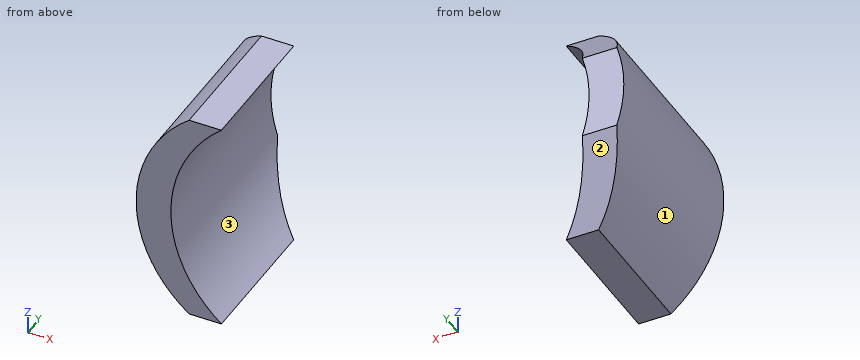
Autodesk Inventor part; units mm, degrees
ref_plane "YZ Plane" through (0, 0, 0) normal (1, 0, 0) x (0, 1, 0)
ref_plane "XZ Plane" through (0, 0, 0) normal (0, 1, 0) x (-1, 0, 0)
ref_plane "XY Plane" through (0, 0, 0) normal (0, 0, 1) x (1, 0, 0)
sketch "Sketch1" plane through (0, 0, 0) normal (0, 1, 0) x (-1, 0, 0)
  arc A0 (0, -6.5) -> (0, 6.5) centre (0, 0) ccw
  line L0 (0, 6.5) -> (0, -6.5)
  dimension "d0" = 13
extrude "Extrusion1" add sketch "Sketch1" along normal blind 12
ref_plane "Work Plane1" through (-10, 0, 6.5) normal (1, 0, 0) x (0, 0, -1)
sketch "Sketch2" plane through (-10, 0, 6.5) normal (1, 0, 0) x (0, 0, -1)
  line L0 (1.5, 8.0057) -> (1.5, 1.5057)
  line L1 (1.5, 1.5057) -> (11.5, 1.5057)
  line L2 (11.5, 1.5057) -> (11.5, 8)
  line L3 (8.5, 10.5) -> (4.5, 10.5)
  line L4 (8.5, 10.5) -> (11.5, 8)
  line L5 (4.5, 10.5) -> (1.5, 8.0057)
  line L6 (13, 0) -> (13, 12)
  point P0 (6.5, 0)
  dimension "d9" = 10
  dimension "d10" = 6.5
  dimension "d12" = 4
  dimension "d14" = 3
  dimension "d15" = 3
  dimension "d24" = 1.5
extrude "Extrusion2" add sketch "Sketch2" along normal blind 10
sketch "Sketch7" plane through (0, 0, 0) normal (0, 1, 0) x (-1, 0, 0)
  arc A0 (0, -6.5) -> (0, 6.5) centre (0, 0) ccw
  line L0 (0, 6.5) -> (0, -6.5)
  line L1 (0, -6.5) -> (0, 6.5)
extrude "Extrusion7" cut sketch "Sketch7" along normal through all
sketch "Sketch8" plane through (0, 0, 0) normal (0, 1, 0) x (-1, 0, 0)
  arc A0 (5.6533, -5) -> (5.6533, 5) centre (1.7994, 0) ccw
  line L0 (5.6533, -5) -> (4.1533, -5)
  line L1 (5.6533, 5) -> (4.1533, 5)
  line L2 (10, 5) -> (4.1533, 5)
  arc A1 (4.1533, -5) -> (4.1533, 5) centre (10.21, 0) ccw
  point P0 (0, 0)
  dimension "d36" = 1.5
  dimension "d37" = 1.5
extrude "Extrusion8" cut sketch "Sketch8" along normal through all both and the other way through all
properties part number "13mm_radius_mold_with_crystal_skull"
CAD build for the part. Positions are in the model's coordinates, mm. Face numbers are marked on the shaded views. Give positions to 0.01 mm unless a question says otherwise; leave off trailing zeros. Order: outer loops, then holes, each group sorted by start corner. A loop starts at its lowest first (then second) coordinate and runs counter-clockwise, first axis right, second up. Notation, with made-up numbers: (65.5, 61.5) - (90.5, 61.5) arc R17 cw to (90.5, 83.5) - close; hole circle Ø9 at (5.5, 74.25). An arc over 180 degrees is marked (long way). Answer in a Markdown table with one row per item.
1. Flat gauge pins, fed straight in: pin 1 (1 mm diameter, centred on x = -6.5, y = 9, fed in from +Z); pin 2 (5 mm diameter, centred on y = 6, z = -4, fed in from -X); pin 3 (5 mm diameter, centred on y = 3, z = -3, fed in from -X). Where does each tip first touch, or does it go through?
Data:
| item | result |
|---|---|
| pin 1 | stops at z = 4.38 |
| pin 2 | stops at x = -7.93 |
| pin 3 | stops at x = -8.09 |
2. Probe probe 1 along Z at (x, y) = (-4.8, 7.75); probe 2 along Z at (x, y) = (-4.55, 4); probe 3 along X at (y, z) = (4.25, -2). List the from-to ranges inside material, lowest first. Write a range as [from, to].
Data:
| item | result |
|---|---|
| probe 1 | z = [-5, -4.38], [4.38, 5] |
| probe 2 | z = [-5, -4.64], [4.64, 5] |
| probe 3 | x = [-7.79, -6.18] |
3. Saw through at D-D, the plane z = 3.25. Give the cut face in (x, y).
Data:
| item | result |
|---|---|
| outline | (-7.21, 1.51) - (-5.63, 1.51) - (-5.63, 9.46) - (-7.21, 9.46) - close |
4. Pull direction Z, two halves, no side cores. Call the marked faces 1, 2 and 3: pulls with the +Z half, pulls with the -Z half, needs draft (parallel to the pull), parting line crosses it, or undercut.
Data:
| item | result |
|---|---|
| face 1 | parting line crosses it |
| face 2 | pulls with the -Z half |
| face 3 | undercut |
5. Saw through at C-C, the plane y = 2. Give the cut face in (x, z), plus the area to 3 significant figures.
Data:
| item | result |
|---|---|
| outline | (-5.65, -5) - (-4.15, -5) arc R6.5 cw to (-4.15, 5) - (-5.65, 5) arc R6.31 ccw to start |
| area | 15.8 mm² |
6. Saw through at B-B, the plane x = -7.6. Give the cut face in (y, z), plus the area to 3 significant figures.
Data:
| item | result |
|---|---|
| outline | (1.51, -2.49) - (10.09, -2.49) - (10.5, -2) - (10.5, 2) - (10.09, 2.49) - (1.51, 2.49) - close |
| area | 44.6 mm² |
7. Saw through at A-A, the plane x = -6.3. Give the cut face in (y, z), plus the area to 3 significant figures.
Data:
| item | result |
|---|---|
| outline | (1.51, -4.43) - (8.48, -4.43) - (10.5, -2) - (10.5, -1.6) - (1.51, -1.6) - close; (1.51, 1.6) - (10.5, 1.6) - (10.5, 2) - (8.48, 4.43) - (1.51, 4.43) - close |
| area | 45.9 mm² |
